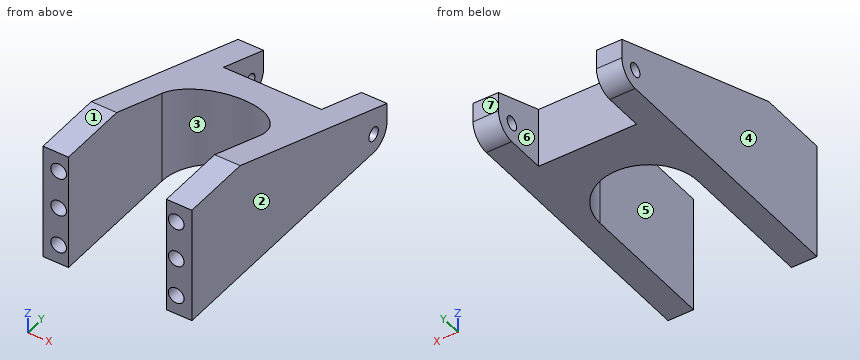
```python
from build123d import *

# Parameters (mm, degrees)
BOSS_EXTRUDE1_DEPTH = 30
SKETCH2_R           = 2
CUT_EXTRUDE1_DEPTH  = 15
FILLET1_R           = 5
CHAMFER1_SIZE       = 20
CHAMFER1_SIZE_2     = 54.949548389
SKETCH3_W           = 25
SKETCH3_H           = 39.596952294
CUT_EXTRUDE2_DEPTH  = 15
SKETCH4_R           = 1.75
CUT_EXTRUDE3_DEPTH  = 62.546730214


with BuildPart() as part:
    # Sketch1 → Boss-Extrude1 (new body)
    with BuildSketch(Plane.XY):
        with BuildLine():
            Line((-12.5, 0), (-12.5, -35))
            Line((-12.5, -35), (-19, -35))
            Line((-19, -35), (-19, 38))
            Line((-19, 38), (19, 38))
            Line((19, 38), (19, -35))
            Line((19, -35), (12.5, -35))
            Line((12.5, -35), (12.5, 0))
            ThreePointArc((12.5, 0), (0, 12.5), (-12.5, 0))
        make_face()
    extrude(amount=BOSS_EXTRUDE1_DEPTH)

    # Sketch2 → Cut-Extrude1 (cut)
    with BuildSketch(Plane.XZ.offset(35)):
        with Locations(Location((-15, 5, 0), (0, 0, 270))):
            Circle(SKETCH2_R)
        with Locations(Location((15, 5, 0), (0, 0, 270))):
            Circle(SKETCH2_R)
        with Locations(Location((-15, 15, 0), (0, 0, 270))):
            Circle(SKETCH2_R)
        with Locations(Location((15, 15, 0), (0, 0, 270))):
            Circle(SKETCH2_R)
        with Locations(Location((-15, 25, 0), (0, 0, 270))):
            Circle(SKETCH2_R)
        with Locations(Location((15, 25, 0), (0, 0, 270))):
            Circle(SKETCH2_R)
    extrude(amount=-CUT_EXTRUDE1_DEPTH, mode=Mode.SUBTRACT)

    # Fillet1
    fillet1_edges = [part.edges().sort_by_distance(p)[0] for p in [
        (0, 38, 0),
    ]]
    fillet(fillet1_edges, radius=FILLET1_R)

    # Chamfer1
    # the kernel refuses this chamfer: 54.949548389, 20 mm, written as the material it takes off along each edge
    with BuildSketch(Plane(origin=(-161.549828987, 38, 30), x_dir=(0, 0.09904090225205052, -0.9950833631817486), z_dir=(1, 0, 0))) as chamfer1_piece_1:
        Polygon((CHAMFER1_SIZE * 0.995083363182, -CHAMFER1_SIZE * 0.0990409022521), (-CHAMFER1_SIZE_2 * 0.0990409022522, -CHAMFER1_SIZE_2 * 0.995083363183), (0, 0), align=None)
    extrude(amount=323.099657974, mode=Mode.SUBTRACT)

    # Sketch3 → Cut-Extrude2 (cut)
    with BuildSketch(Plane(origin=(0, 38, 0), x_dir=(1, 0, 0), z_dir=(0, 1, 0))):
        Rectangle(SKETCH3_W, SKETCH3_H)
    extrude(amount=-CUT_EXTRUDE2_DEPTH, mode=Mode.SUBTRACT)

    # Sketch4 → Cut-Extrude3 (cut, through all)
    with BuildSketch(Plane.ZY.offset(19)):
        with Locations((5, 33)):
            Circle(SKETCH4_R)
    extrude(amount=-CUT_EXTRUDE3_DEPTH, mode=Mode.SUBTRACT)


solid = part.part
```
The model under review builds one solid part; all positions refer to its coordinate system, in mm. Face numbers are marked on the shaded views. A direction names the side the tool comes from. Give positions to 0.01 mm unless a question says otherwise; leave off trailing zeros. Write each loop counter-clockwise with the first axis right and the second up, starting at its lowest first coordinate (ties: lowest second). Pieces come first, ordered by that corner, then holes.
(1) Consider section D-D, the plane y = -15. Give the boundary of the cut face in (x, z).
(2) Consider section A-A, the plane z = 25. Give the boundary of the cut face in (x, y).
(3) Consider section C-C, the plane z = 8. Give the boundary of the cut face in (x, y).
(4) The part is to be moulded in two halves that separate along X. For the marked faces 1, 2, 3 and 4, say which applies: released by +X, released by -X, zero draft, split by the parting line, or undercut.
(5) Tool access review of the marked faces 5, 6 and 7: name each direction out of +Z, -Z, +X, -X, +Y, -Y from which nothing blocks a thin tool from reaching the whole face with its end or side.
(6) For P1, Ø2, axis at y = 33, z = 5, coming from the +X side; P2, Ø2, axis at x = 8, z = 7.5, coming from the -Y side; P3, Ø4.5, axis at x = 15, z = 5, coming from the -Y side; P4, Ø12, axis at x = -2.5, z = 12.5, coming from the -Y side, all flat-tipped, find the tip position at first contact; note any pin that passes through.
(7) Consider section B-B, the plane x = 15. Give the boundary of the cut face in (y, z).
(8) To check wall thickness, follow L1, parallel to X at y = -29, z = 5; L2, parallel to X at y = 27.5, z = 9.5; L3, parallel to Y at x = 14.5, z = 5. State the ranges of each line that lie inside material, in increasing order.
Returned:
1. outline: (-19, 0) - (-12.5, 0) - (-12.5, 29.29) - (-19, 29.29) - close; (12.5, 0) - (19, 0) - (19, 29.29) - (12.5, 29.29) - close
2. outline: (-19, -35) - (-17, -35) - (-17, -20) - (-13, -20) - (-13, -35) - (-12.5, -35) - (-12.5, -3.21) - (-19, -3.21) - close; (12.5, -35) - (13, -35) - (13, -20) - (17, -20) - (17, -35) - (19, -35) - (19, -3.21) - (12.5, -3.21) - close
3. outline: (-19, -35) - (-12.5, -35) - (-12.5, 0) arc R12.5 cw to (12.5, 0) - (12.5, -35) - (19, -35) - (19, 38) - (12.5, 38) - (12.5, 23) - (-12.5, 23) - (-12.5, 38) - (-19, 38) - close
4. face 1: zero draft
4. face 2: released by +X
4. face 3: undercut
4. face 4: released by -X
5. face 5: +Z, -Z, -Y
5. face 6: +Z, -Z, +Y
5. face 7: +Z, -Z, +X, -X, +Y
6. P1: passes through
6. P2: stops at y = 8.67
6. P3: stops at y = -35
6. P4: stops at y = 9.17
7. outline: (-35, 0) - (33, 0) arc R5 ccw to (38, 5) - (38, 10) - (-16.95, 30) - (-35, 30) - (-35, 27) - (-20, 27) - (-20, 23) - (-35, 23) - (-35, 17) - (-20, 17) - (-20, 13) - (-35, 13) - (-35, 7) - (-20, 7) - (-20, 3) - (-35, 3) - close; hole circle Ø3.5 at (33, 5)
8. L1: x = -19 to -17, -13 to -12.5, 12.5 to 13, 17 to 19
8. L2: x = -19 to -12.5, 12.5 to 19
8. L3: y = -20 to 31.25, 34.75 to 38
